Model file for the job. Use its own axes, mm. A direction names the side the tool comes from. Round coordinates to 2 decimals unless told otherwise and drop trailing zeros. Order: outer loops, then holes, each group sorted by start corner. A loop starts at its lowest first (then second) coordinate and runs counter-clockwise, first axis right, second up. Notation, with made-up numbers: (25, 13.25) -> (48, 13.25) arc R6 ccw to (48, 23.25) -> close; hole circle Ø4 at (-28, 74). An arc over 180 degrees is marked (long way). Use CSV: the item, a comma, the result in double quotes.
```python
from build123d import *

# Parameters (mm, degrees)
ESQUISSE1_R               = 2.5
EXTRUSION1_DEPTH          = 5
TROU_TARAUD_M3X0_51_D     = 2.5
TROU_TARAUD_M3X0_51_DEPTH = 9.1
TROU_TARAUD_M3X0_51_TIP   = 0.751075774


with BuildPart() as part:
    # Esquisse1 → Extrusion1 (new body)
    with BuildSketch(Plane.XY):
        with BuildLine():
            Line((-19.5, 10), (-19.5, -20))
            Line((-19.5, -20), (3.888568512, -6.991354299))
            ThreePointArc((3.888568512, -6.991354299), (7.834576447, 1.618459728), (0.799950986, 7.959904423))
            Line((0.799950986, 7.959904423), (-19.5, 10))
        make_face()
        Circle(ESQUISSE1_R, mode=Mode.SUBTRACT)
    extrude(amount=EXTRUSION1_DEPTH)

    # Trou taraudé M3x0.51
    with Locations(Plane.ZY.offset(19.5)):
        with Locations((2.5, 6), (2.5, -16)):
            Hole(TROU_TARAUD_M3X0_51_D / 2, depth=TROU_TARAUD_M3X0_51_DEPTH)
            with Locations((0, 0, -(TROU_TARAUD_M3X0_51_DEPTH + TROU_TARAUD_M3X0_51_TIP / 2))):  # 118° drill point
                Cone(0, TROU_TARAUD_M3X0_51_D / 2, TROU_TARAUD_M3X0_51_TIP, mode=Mode.SUBTRACT)


solid = part.part
```
Q1. Which spindle directions (+Z, -Z, +X, -X, +Y, -Y) get a long thin tool onto all of the face, cutting with end or side? Do faces 4 (the cylindrical face through (-15.9, -14.76, 2.66)), 5 (the cylindrical face through (-0.54, -2.44, 2.46)). Say none if no direction does.
From the geometry:
face 4,"-X"
face 5,"+Z, -Z"
Q2. Mould opens along Z. For faces 1 (the flat face through (-9, -1, 0)), 2 (the cylindrical face through (7.86, 1.48, 2.46)), 3 (the cylindrical face through (-14.886, 4.891, 1.923)) say: +Z half, -Z half, draft (parallel to the pull), parting line (faces both ways), or undercut.
From the geometry:
face 1,"-Z half"
face 2,"draft"
face 3,"undercut"
Q3. Cut at A-A (y = -16). Give the cut face in (x, z).
From the geometry:
outline,"(-19.5, 0) -> (-12.31, 0) -> (-12.31, 1.25) -> (-19.5, 1.25) -> close; (-19.5, 3.75) -> (-12.31, 3.75) -> (-12.31, 5) -> (-19.5, 5) -> close"
Q4. Cut at B-B (z = 4.35). Give the cut face in (x, y), plus the area to 3 significant figures.
From the geometry:
outline,"(-19.5, -20) -> (3.89, -6.99) arc R8 ccw to (0.8, 7.96) -> (-19.5, 10) -> close; hole circle Ø5 at (0, 0)"
area,"543 mm²"
Q5. Cut at C-C (x = 0). Give the cut face in (y, z), plus the area to 3 significant figures.
From the geometry:
outline,"(-9.15, 0) -> (-2.5, 0) -> (-2.5, 5) -> (-9.15, 5) -> close; (2.5, 0) -> (8.04, 0) -> (8.04, 5) -> (2.5, 5) -> close"
area,"61.0 mm²"
Q6. Pin check, flat tips, straight feed: pin 1 (3 mm diameter, centred on y = 6, z = 2.5, fed in from +X); pin 2 (3 mm diameter, centred on y = 4.5, z = 3, fed in from +X); pin 3 (3 mm diameter, centred on x = -4.5, z = 3.5, fed in from +Y). Stop position of each tip, or through.
From the geometry:
pin 1,"stops at x = 6.61"
pin 2,"stops at x = 7.42"
pin 3,"stops at y = 8.64"
Q7. Cut at D-D (x = -16.5). Give the cut face in (y, z), plus the area to 3 significant figures.
From the geometry:
outline,"(-18.33, 0) -> (9.7, 0) -> (9.7, 5) -> (-18.33, 5) -> close; hole circle Ø2.5 at (-16, 2.5); hole circle Ø2.5 at (6, 2.5)"
area,"130 mm²"
Q8. Probe line 1 along Y through (x, z) = (-15.75, 2.5); line 2 along Y through (x, z) = (-16.25, 2.5); line 3 along Z through (x, y) = (-17, -16). List the from-to ranges inside material, lowest first.
From the geometry:
line 1,"y = -17.91 to -17.25, -14.75 to 4.75, 7.25 to 9.62"
line 2,"y = -18.19 to -17.25, -14.75 to 4.75, 7.25 to 9.67"
line 3,"z = 0 to 1.25, 3.75 to 5"
